from build123d import *

# Parameters (mm, degrees)
F0_R     = 12.5
F0_R_2   = 12
F1_DEPTH = 5.4
F2_R     = 12.5
F3_DEPTH = 1
F4_R     = 12.5
F4_R_2   = 10.1
F5_DEPTH = 4


with BuildPart() as f1:
    # F0 (on Top) → F1 (new body)
    with BuildSketch(Plane.XY):
        Circle(F0_R)
        Circle(F0_R_2, mode=Mode.SUBTRACT)
    extrude(amount=F1_DEPTH)

    # F2 (on Top) → F3 (join)
    with BuildSketch(Plane.XY):
        Circle(F2_R)
    extrude(amount=F3_DEPTH)

    # F4 (on Top) → F5 (join)
    with BuildSketch(Plane.XY):
        Circle(F4_R)
        Circle(F4_R_2, mode=Mode.SUBTRACT)
    extrude(amount=F5_DEPTH)


solid = f1.part
Can you work these out from the model? Positions are in its coordinate system, mm. A direction names the side the tool comes from. Coordinates: 2 decimals unless noted, no trailing zeros. Order: outer loops, then holes, each group sorted by start corner. A loop starts at its lowest first (then second) coordinate and runs counter-clockwise, first axis right, second up. Notation, with made-up numbers: M 21.5,23.5 L 48.5,23.5 A16 ccw 48.5,49.5 Z; hole C -16.75,58.25 d10. An arc over 180 degrees is marked long. Answer as CSV lines item,"result".
(1) If we mould it in two halves opening along X, with no side actions, what happens to faces 3 (the cylindrical face through (-11.99, 0.53, 4.69)), 4 (the cylindrical face through (11.923, 3.755, 2.662)), 5 (the flat face through (0, 0, 0))? For each: released by +X, released by -X, zero draft, split by the parting line, or undercut.
Geometry check:
face 3,"undercut"
face 4,"split by the parting line"
face 5,"zero draft"
(2) Suppose I cut it at C-C on z = 1.8. Please give me the cut outline in (x, y), plus the area to 3 significant figures.
Geometry check:
outline,"C 0,0 d25; hole C 0,0 d20.2"
area,"170 mm^2"
(3) I'm going to push flat-ended pins straight in: pin 1 (6 mm diameter, centred on x = 3.5, y = -5.5, fed in from +Z); pin 2 (3 mm diameter, centred on x = 4.5, z = 4.5, fed in from -Y); pin 3 (12 mm diameter, centred on x = 0, y = 0, fed in from -Z); pin 4 (8 mm diameter, centred on x = 5.5, y = 4.5, fed in from +Z). Where does each tip first touch, or does it pass through?
Geometry check:
pin 1,"z = 1"
pin 2,"y = -12.13"
pin 3,"z = 0"
pin 4,"z = 4"
(4) Suppose I cut it at D-D on x = 11. Please give me the cut outline in (y, z).
Geometry check:
outline,"M -5.94,0 L 5.94,0 L 5.94,5.4 L 4.8,5.4 L 4.8,4 L -4.8,4 L -4.8,5.4 L -5.94,5.4 Z"
(5) Please list where these lines run through material, in increasing order: L1, parallel to Y at x = 0, z = 2.5; L2, parallel to Z at x = 0.75, y = -7.5.
Geometry check:
L1,"-12.5 to -10.1, 10.1 to 12.5"
L2,"0 to 1"
(6) On a 3-axis mill with a long thin cutter (end or side, diameter ignored), from which of +Z, -Z, +X, -X, +Y, -Y can I reach the whole of each face in a straight line? I mean faces 1 (the flat face through (0, 0, 1)), 2 (the flat face through (-7, 10, 5.4)). Say none if no direction works.
Geometry check:
face 1,"+Z"
face 2,"+Z, +X, -X, +Y, -Y"
(7) Suppose I cut it at A-A on x = 0. Please give me the cut outline in (y, z).
Geometry check:
outline,"M -12.5,0 L 12.5,0 L 12.5,5.4 L 12,5.4 L 12,4 L 10.1,4 L 10.1,1 L -10.1,1 L -10.1,4 L -12,4 L -12,5.4 L -12.5,5.4 Z"
